Work out the finished part from the listing and answer in its coordinate system (mm). A direction names the side the tool comes from. Give positions to 0.01 mm unless a question says otherwise; leave off trailing zeros. Order: outer loops, then holes, each group sorted by start corner. A loop starts at its lowest first (then second) coordinate and runs counter-clockwise, first axis right, second up. Notation, with made-up numbers: (-3.5, -10.5) -> (14.5, -10.5) arc R19 ccw to (14.5, 5.5) -> close; hole circle Ø2 at (-34, 83). An arc over 180 degrees is marked (long way). Answer as CSV lines item,"result". Start each with the question number.
1. A cutting plane is placed at D-D (x = 220). Give the vertices of the cut face in (y, z).
2. A cutting plane is placed at C-C (y = -88). Give the vertices of the cut face in (x, z), then the cut area to 3 significant figures.
3. For a pull along X with two mould halves and no side action, classify faces 4 (the cylindrical face through (-190.42, 13.38, 16.28)), 5 (the cylindrical face through (44.406, -50.75, 16.279)), 6 (the flat face through (-1, 21, 0)), 7 (the cylindrical face through (143.427, 258.227, 16.279)) as released by +X, released by -X, zero draft, split by the parting line, or undercut.
4. A cutting plane is placed at A-A (x = 95). Give the vertices of the cut face in (y, z).
5. Find the intervals of material crossed by L1, parallel to Y at x = -124, z = 7; L2, parallel to Y at x = 129.5, z = 30.5; L3, parallel to Y at x = 192, z = 29, in increasing order.
6. For faces 1 (the cylindrical face through (101.843, -255.997, 16.279)), 2 (the flat face through (-221.39, -34.67, 16.28)), 3 (the flat face through (177.276, 2.292, 16.279)), determine the directions among +Z, -Z, +X, -X, +Y, -Y from which every point of the face is accessible in a straight line to the end or side of a thin tool.
7. Flat-ended cylindrical pins translate along their axes: pin 1 (8 mm diameter, centred on x = 86, z = 15.5, fed in from -Y); pin 2 (1.5 mm diameter, centred on x = 88.5, z = 13, fed in from -Y); pin 3 (1.5 mm diameter, centred on y = -106.5, z = 7.5, fed in from +X). Find the tip coordinate at first contact, or state that the pin passes through.
8. A cutting plane is placed at B-B (y = 160). Give the vertices of the cut face in (x, z).
from build123d import *

# Parameters (mm, degrees)
F2_R     = 111.219822
F2_R_2   = 107.971154
F3_DEPTH = 33.02
F4_R     = 168.535103


with BuildPart() as f3:
    # F2 (on Top) → F3 (new body)
    with BuildSketch(Plane.XY):
        with BuildLine():
            ThreePointArc((-230.728179, -44.370614), (-251.440516, -82.851948), (-258.738101, -125.939757))
            ThreePointArc((-258.738101, -125.939757), (-219.839177, -219.580253), (-126.260236, -258.627027))
            ThreePointArc((-126.260236, -258.627027), (-102.176368, -256.061677), (-78.85915, -249.510258))
            ThreePointArc((-78.85915, -249.510258), (-29.568087, -216.546357), (0, -165.146396))
            ThreePointArc((0, -165.146396), (29.560129, -216.553795), (78.85915, -249.510258))
            ThreePointArc((78.85915, -249.510258), (102.176368, -256.061677), (126.260236, -258.627027))
            ThreePointArc((126.260236, -258.627027), (219.839177, -219.580253), (258.738101, -125.939757))
            ThreePointArc((258.738101, -125.939757), (251.440516, -82.851948), (230.728179, -44.370614))
            Line((230.728179, -44.370614), (212.309614, -25.240019))
            ThreePointArc((212.309614, -25.240019), (194.800133, -12.709117), (175.517112, -3.129424))
            Line((175.517112, -3.129424), (179.085225, 7.86738))
            ThreePointArc((179.085225, 7.86738), (190.270178, 13.298483), (200.912178, 19.728716))
            Line((200.912178, 19.728716), (229.211181, 45.454361))
            ThreePointArc((229.211181, 45.454361), (251.18703, 84.187969), (258.738101, 128.076598))
            ThreePointArc((258.738101, 128.076598), (140.740138, 258.514188), (0, 153.016806))
            ThreePointArc((0, 153.016806), (-140.740138, 258.514188), (-258.738101, 128.076598))
            ThreePointArc((-258.738101, 128.076598), (-251.18703, 84.187969), (-229.211181, 45.454361))
            Line((-229.211181, 45.454361), (-200.912178, 19.728716))
            ThreePointArc((-200.912178, 19.728716), (-190.270178, 13.298483), (-179.085225, 7.86738))
            Line((-179.085225, 7.86738), (-175.517112, -3.129424))
            ThreePointArc((-175.517112, -3.129424), (-194.800133, -12.709117), (-212.309614, -25.240019))
            Line((-212.309614, -25.240019), (-230.728179, -44.370614))
        make_face()
        with Locations((-126.379907, -125.917777)):
            Circle(F2_R, mode=Mode.SUBTRACT)
        with Locations((126.379907, -125.917777)):
            Circle(F2_R, mode=Mode.SUBTRACT)
        with Locations((-128.127411, 128.015205)):
            Circle(F2_R_2, mode=Mode.SUBTRACT)
        with Locations((128.127411, 128.015205)):
            Circle(F2_R_2, mode=Mode.SUBTRACT)
    extrude(amount=F3_DEPTH)

    # F4
    f4_edges = [f3.edges().sort_by_distance(p)[0] for p in [
        (0, -165.146396, 16.51),
    ]]
    fillet(f4_edges, radius=F4_R)


solid = f3.part
Answer sheet:
1,outline,"(-219.42, 0) -> (-185.96, 0) -> (-185.96, 33.02) -> (-219.42, 33.02) -> close; (-65.88, 0) -> (-33.23, 0) -> (-33.23, 33.02) -> (-65.88, 33.02) -> close; (37.08, 0) -> (71.29, 0) -> (71.29, 33.02) -> (37.08, 33.02) -> close; (184.74, 0) -> (221.39, 0) -> (221.39, 33.02) -> (184.74, 33.02) -> close"
2,outline,"(-253.09, 0) -> (-230.94, 0) -> (-230.94, 33.02) -> (-253.09, 33.02) -> close; (-21.82, 0) -> (21.82, 0) -> (21.82, 33.02) -> (-21.82, 33.02) -> close; (230.94, 0) -> (253.09, 0) -> (253.09, 33.02) -> (230.94, 33.02) -> close"
2,area,"2,900 mm^2"
3,face 4,"released by -X"
3,face 5,"undercut"
3,face 6,"zero draft"
3,face 7,"undercut"
4,outline,"(-254.49, 0) -> (-232.62, 0) -> (-232.62, 33.02) -> (-254.49, 33.02) -> close; (-19.22, 0) -> (25.25, 0) -> (25.25, 33.02) -> (-19.22, 33.02) -> close; (230.78, 0) -> (254.82, 0) -> (254.82, 33.02) -> (230.78, 33.02) -> close"
5,L1,"y = -258.56 to -237.11, -14.72 to 20.12, 235.91 to 259.05"
5,L2,"y = -258.57 to -237.09, -14.74 to 20.05, 235.98 to 259.11"
5,L3,"y = -240.92 to -215.72, -36.12 to -11.07, 14.25 to 40.96, 215.07 to 242.47"
6,face 1,"+Z, -Z, -Y"
6,face 2,"+Z, -Z, -X"
6,face 3,"+Z, -Z, +X"
7,pin 1,"stops at y = -253.17"
7,pin 2,"stops at y = -252.95"
7,pin 3,"stops at x = 257.34"
8,outline,"(-254.9, 0) -> (-231.25, 0) -> (-231.25, 33.02) -> (-254.9, 33.02) -> close; (-25, 0) -> (-1.53, 0) -> (-1.53, 33.02) -> (-25, 33.02) -> close; (1.53, 0) -> (25, 0) -> (25, 33.02) -> (1.53, 33.02) -> close; (231.25, 0) -> (254.9, 0) -> (254.9, 33.02) -> (231.25, 33.02) -> close"
